```python
from build123d import *

# Parameters (mm, degrees)
SKETCH_1_R                   = 18.4
EXTRUDE_1_DEPTH              = 21.5
SKETCH_2_R                   = 6
EXTRUDE_2_DEPTH              = 6
SKETCH_3_R                   = 3
EXTRUDE_3_DEPTH              = 16
SKETCH_4_W                   = 5
SKETCH_4_H                   = 1
CUT_EXTRUDE_1_DEPTH          = 11.85
SKETCH_5_R                   = 17.4
EXTRUDE_4_DEPTH              = 30.7
SKETCH_6_R                   = 17
EXTRUDE_5_DEPTH              = 15.4
CUT_EXTRUDE_START            = 15
SKETCH_7_W                   = 13.6
SKETCH_7_H                   = 3.8
CUT_EXTRUDE_2_DEPTH          = 58.435350486
SKETCH_8_R                   = 0.6
EXTRUDE_6_DEPTH              = 5
HOLE_WIZARD_M3_1_D           = 2.5
HOLE_WIZARD_M3_1_DEPTH       = 8.5
HOLE_WIZARD_M3_1_CSINK_D     = 3.05
HOLE_WIZARD_M3_1_CSINK_ANGLE = 90
HOLE_WIZARD_M3_1_TIP         = 0.751075774
CUT_EXTRUDE_3_DEPTH          = 0.3


with BuildPart() as part:
    # 草图1 → 凸台-拉伸1 (new body)
    with BuildSketch(Plane(origin=(0, 0, 0), x_dir=(1, 0, 0), z_dir=(0, 1, 0))):
        with Locations(Location((0, 0, 0), (0, 0, 270))):
            Circle(SKETCH_1_R)
    extrude(amount=-EXTRUDE_1_DEPTH)

    # 草图2 → 凸台-拉伸2 (add)
    with BuildSketch(Plane(origin=(0, 0, 0), x_dir=(1, 0, 0), z_dir=(0, 1, 0))):
        with Locations(Location((0, -7, 0), (0, 0, 270))):
            Circle(SKETCH_2_R)
    extrude(amount=EXTRUDE_2_DEPTH)

    # 草图3 → 凸台-拉伸3 (add)
    with BuildSketch(Plane(origin=(0, 6, 0), x_dir=(1, 0, 0), z_dir=(0, 1, 0))):
        with Locations(Location((0, -7, 0), (0, 0, 270))):
            Circle(SKETCH_3_R)
    extrude(amount=EXTRUDE_3_DEPTH)

    # 草图4 → 切除-拉伸1 (cut)
    with BuildSketch(Plane(origin=(0, 22, 0), x_dir=(1, 0, 0), z_dir=(0, 1, 0))):
        with Locations((0, -4.1)):
            Rectangle(SKETCH_4_W, SKETCH_4_H)
    extrude(amount=-CUT_EXTRUDE_1_DEPTH, mode=Mode.SUBTRACT)

    # 草图5 → 凸台-拉伸4 (add)
    with BuildSketch(Plane.XZ.offset(21.5)):
        with Locations(Location((0, 0, 0), (0, 0, 90))):
            Circle(SKETCH_5_R)
    extrude(amount=EXTRUDE_4_DEPTH)

    # 草图6 → 凸台-拉伸5 (add)
    with BuildSketch(Plane.XZ.offset(52.2)):
        with Locations(Location((0, 0, 0), (0, 0, 90))):
            Circle(SKETCH_6_R)
    extrude(amount=EXTRUDE_5_DEPTH)

    # 草图7 → 切除-拉伸2 (cut, through all)
    with BuildSketch(Plane.XY.offset(CUT_EXTRUDE_START)):
        with Locations((0, -56.6)):
            Rectangle(SKETCH_7_W, SKETCH_7_H)
    extrude(amount=CUT_EXTRUDE_2_DEPTH, mode=Mode.SUBTRACT)

    # 草图8 → 凸台-拉伸6 (add)
    with BuildSketch(Plane.XY.offset(15)):
        with Locations((-5, -56.6)):
            Circle(SKETCH_8_R)
        with Locations((-3, -56.6)):
            Circle(SKETCH_8_R)
        with Locations((-1, -56.6)):
            Circle(SKETCH_8_R)
        with Locations(Location((1, -56.6, 0), (0, 0, 180))):
            Circle(SKETCH_8_R)
        with Locations(Location((3, -56.6, 0), (0, 0, 180))):
            Circle(SKETCH_8_R)
        with Locations(Location((5, -56.6, 0), (0, 0, 180))):
            Circle(SKETCH_8_R)
    extrude(amount=EXTRUDE_6_DEPTH)

    # M3 螺纹孔1
    with Locations(Plane(origin=(0, 0, 0), x_dir=(1, 0, 0), z_dir=(0, 1, 0))):
        with Locations((-7.75, 13.423393759), (15.5, 0), (7.75, -13.423393759), (-7.75, -13.423393759), (-15.5, 0), (7.75, 13.423393759)):
            CounterSinkHole(HOLE_WIZARD_M3_1_D / 2, HOLE_WIZARD_M3_1_CSINK_D / 2, depth=HOLE_WIZARD_M3_1_DEPTH, counter_sink_angle=HOLE_WIZARD_M3_1_CSINK_ANGLE)
            with Locations((0, 0, -(HOLE_WIZARD_M3_1_DEPTH + HOLE_WIZARD_M3_1_TIP / 2))):  # 118° drill point
                Cone(0, HOLE_WIZARD_M3_1_D / 2, HOLE_WIZARD_M3_1_TIP, mode=Mode.SUBTRACT)

    # 草图12 → 切除-拉伸3 (cut)
    with BuildSketch(Plane(origin=(0, 0, 0), x_dir=(1, 0, 0), z_dir=(0, 1, 0))):
        with BuildLine():
            ThreePointArc((7.687453335, -9.214285714), (0, 12), (-7.687453335, -9.214285714))
            ThreePointArc((-7.687453335, -9.214285714), (0, 1), (7.687453335, -9.214285714))
        make_face()
    extrude(amount=-CUT_EXTRUDE_3_DEPTH, mode=Mode.SUBTRACT)


solid = part.part
```
Geometry check sheet. Reference: the model listing, model coordinates, mm. A direction names the side the tool comes from. Coordinates: 2 decimals unless noted, no trailing zeros. Order: outer loops, then holes, each group sorted by start corner. A loop starts at its lowest first (then second) coordinate and runs counter-clockwise, first axis right, second up.
Item 1: Section check B-B (z = -4.5). Enter the section's corners in (x, y).
Item 2: Depth check by flat-ended pin: pin 1 (3 mm diameter, centred on y = -41.5, z = -5, fed in from -X); pin 2 (2 mm diameter, centred on x = 7.75, z = -13.42, fed in from +Y); pin 3 (4 mm diameter, centred on x = -7.75, z = -13.42, fed in from +Y). Enter the tip coordinate at first touch or a pass-through.
Item 3: Tool access check on faces 1 (the flat face through (0, -58.5, 16)), 2 (the flat face through (0, -67.6, 0)), 3 (the cylindrical face through (8.67, -4.45, 12.58)). Record the directions out of +Z, -Z, +X, -X, +Y, -Y that give a thin tool (end or side, any length) a straight path to the whole face; none if there is none.
Item 4: Section check C-C (y = -31.5). Enter the section's corners in (x, z), plus the area to 3 significant figures.
Item 5: Scan lines: line 1 along Z through (x, y) = (7.75, -2); line 2 along Y through (x, z) = (14, -6); line 3 along Z through (x, y) = (-7, -3). Record each from-to range of solid material in increasing order.
Item 6: Mould release check, pull along Z, two halves, no side actions. Record for faces 4 (the cylindrical face through (-1.15, 13.89, 9.77)), 5 (the flat face through (11, -21.5, 14)), 6 (the cylindrical face through (-14.25, -4.45, -0.05)), 7 (the cylindrical face through (16.75, -4.45, -0.05)): released by +Z, released by -Z, zero draft, split by the parting line, or undercut.
Item 7: Section check A-A (x = 13). Enter the section's corners in (y, z), plus the area to 3 significant figures.
Check sheet entries:
1. outline: (-17.84, -21.5) - (-16.81, -21.5) - (-16.81, -52.2) - (-16.39, -52.2) - (-16.39, -67.6) - (16.39, -67.6) - (16.39, -52.2) - (16.81, -52.2) - (16.81, -21.5) - (17.84, -21.5) - (17.84, 0) - (11.12, 0) - (11.12, -0.3) - (-11.12, -0.3) - (-11.12, 0) - (-17.84, 0) - close
2. pin 1: stops at x = -17.04
2. pin 2: stops at y = -8.65
2. pin 3: stops at y = 0
3. face 1: +Z
3. face 2: +Z, -Z, +X, -X, -Y
3. face 3: +Y
4. outline: circle Ø34.8 at (0, 0)
4. area: 951 mm2
5. line 1: z = -16.69 to -14.67, -12.17 to 12.17, 14.67 to 16.69
5. line 2: y = -67.6 to 0
5. line 3: z = -17.02 to -14.42, -12.42 to 12.42, 14.42 to 17.02
6. face 4: split by the parting line
6. face 5: zero draft
6. face 6: undercut
6. face 7: undercut
7. outline: (-67.6, -10.95) - (-52.2, -10.95) - (-52.2, -11.57) - (-21.5, -11.57) - (-21.5, -13.02) - (0, -13.02) - (0, 13.02) - (-21.5, 13.02) - (-21.5, 11.57) - (-52.2, 11.57) - (-52.2, 10.95) - (-67.6, 10.95) - close
7. area: 1,610 mm2
